from build123d import *

# Parameters (mm, degrees)
BOSS_EXTRUDE1_DEPTH = 19.5
BOSS_EXTRUDE5_DEPTH = 1.5
BOSS_EXTRUDE6_DEPTH = 1.5
SKETCH8_R           = 6.75
CUT_EXTRUDE2_DEPTH  = 35.70752685
BOSS_EXTRUDE7_DEPTH = 2.5
SKETCH10_R          = 1.75
BOSS_EXTRUDE8_DEPTH = 5
CHAMFER1_SIZE       = 1.5
SKETCH11_R          = 1.75
CUT_EXTRUDE3_DEPTH  = 3
CHAMFER2_SIZE       = 1
REVOLVE1_ANGLE      = 180


with BuildPart() as part:
    # Sketch1 → Boss-Extrude1 (new body)
    with BuildSketch(Plane.XY):
        Polygon((-11.779, -12.684829289), (-10.279, -12.684829289), (-10.279, -0.473504424), (-11.944063509, 0.487820441), (-11.944063509, 1.64252098), (-9.912974596, 2.815170711), (-9.427494989, 2.815170711), (-9.427494989, 4.973204454), (-6.75, 9.910826582), (0, 9.910826582), (0, 12.684829289), (-7.456216647, 12.684829289), (-13.444063509, 1.64252098), (-13.444063509, 0.487820441), align=None)
    extrude(amount=BOSS_EXTRUDE1_DEPTH)

    # Sketch6 → Boss-Extrude5 (add)
    with BuildSketch(Plane.XY.offset(19.5)):
        Polygon((0, 12.684829289), (-7.456216647, 12.684829289), (-13.444063509, 1.64252098), (-13.444063509, 0.487820441), (-11.779, -12.684829289), (0, -12.684829289), align=None)
    extrude(amount=-BOSS_EXTRUDE5_DEPTH)

    # Sketch7 → Boss-Extrude6 (add)
    with BuildSketch(Plane(origin=(0, 0, 0), x_dir=(-1, 0, 0), z_dir=(0, 0, -1))):
        Polygon((0, 12.684829289), (0, -12.684829289), (11.779, -12.684829289), (13.444063509, 0.487820441), (13.444063509, 1.64252098), (7.456216647, 12.684829289), align=None)
    extrude(amount=-BOSS_EXTRUDE6_DEPTH)

    # Sketch8 → Cut-Extrude2 (cut, through all)
    with BuildSketch(Plane(origin=(0, 12.684829289, 0), x_dir=(1, 0, 0), z_dir=(0, 1, 0))):
        with Locations((0, -9.75)):
            Circle(SKETCH8_R)
    extrude(amount=-CUT_EXTRUDE2_DEPTH, mode=Mode.SUBTRACT)

    # Sketch9 → Boss-Extrude7 (add, symmetric)
    with BuildSketch(Plane(origin=(0, 12.684829289, 0), x_dir=(1, 0, 0), z_dir=(0, 1, 0))):
        with BuildLine():
            Line((0, -1.5), (0, -3))
            ThreePointArc((0, -3), (-6.75, -9.75), (0, -16.5))
            Line((0, -16.5), (0, -18))
            ThreePointArc((0, -18), (-8.25, -9.75), (0, -1.5))
        make_face()
    extrude(amount=BOSS_EXTRUDE7_DEPTH, both=True)

    # Sketch10 → Boss-Extrude8 (add)
    with BuildSketch(Plane(origin=(0, 0, 0), x_dir=(0, 0, -1), z_dir=(1, 0, 0))):
        Polygon((-19.5, 12.684829289), (-27.043783602, 4.79693847), (-27.043783602, -4.79693847), (-19.5, -12.684829289), align=None)
        Polygon((-20.396891801, -1.659882024), (-20.396891801, 1.659882024), (-23.271891801, 3.319764048), (-26.146891801, 1.659882024), (-26.146891801, -1.659882024), (-23.271891801, -3.319764048), align=None, mode=Mode.SUBTRACT)
        Polygon((-23.271891801, -3.319764048), (-20.396891801, -1.659882024), (-20.396891801, 1.659882024), (-23.271891801, 3.319764048), (-26.146891801, 1.659882024), (-26.146891801, -1.659882024), align=None)
        with Locations(Location((-23.271891801, 0, 0), (0, 0, 90))):
            Circle(SKETCH10_R, mode=Mode.SUBTRACT)
        Polygon((7.543783602, 4.79693847), (0, 12.684829289), (0, -12.684829289), (7.543783602, -4.79693847), align=None)
        Polygon((6.646891801, 1.659882024), (3.771891801, 3.319764048), (0.896891801, 1.659882024), (0.896891801, -1.659882024), (3.771891801, -3.319764048), (6.646891801, -1.659882024), align=None, mode=Mode.SUBTRACT)
        Polygon((6.646891801, 1.659882024), (6.646891801, -1.659882024), (3.771891801, -3.319764048), (0.896891801, -1.659882024), (0.896891801, 1.659882024), (3.771891801, 3.319764048), align=None)
        with Locations(Location((3.771891801, 0, 0), (0, 0, 90))):
            Circle(SKETCH10_R, mode=Mode.SUBTRACT)
    extrude(amount=-BOSS_EXTRUDE8_DEPTH)

    # Chamfer1
    chamfer1_edges = [part.edges().sort_by_distance(p)[0] for p in [
        (-12.611531755, -6.098504424, 19.5),
        (-13.444063509, 1.065170711, 19.5),
        (-10.450140078, 7.163675135, 19.5),
        (-12.611531755, -6.098504424, 0),
        (-13.444063509, 1.065170711, 0),
        (-10.450140078, 7.163675135, 0),
    ]]
    chamfer(chamfer1_edges, length=CHAMFER1_SIZE)

    # Sketch11 → Cut-Extrude3 (cut)
    with BuildSketch(Plane.ZY.offset(5)):
        Polygon((-6.646891801, 1.659882024), (-3.771891801, 3.319764048), (-0.896891801, 1.659882024), (-0.896891801, -1.659882024), (-3.771891801, -3.319764048), (-6.646891801, -1.659882024), align=None)
        with Locations(Location((-3.771891801, 0, 0), (0, 0, 90))):
            Circle(SKETCH11_R, mode=Mode.SUBTRACT)
        Polygon((20.396891801, 1.659882024), (23.271891801, 3.319764048), (26.146891801, 1.659882024), (26.146891801, -1.659882024), (23.271891801, -3.319764048), (20.396891801, -1.659882024), align=None)
        with Locations(Location((23.271891801, 0, 0), (0, 0, 90))):
            Circle(SKETCH11_R, mode=Mode.SUBTRACT)
    extrude(amount=-CUT_EXTRUDE3_DEPTH, mode=Mode.SUBTRACT)

    # Chamfer2
    chamfer2_edges = [part.edges().sort_by_distance(p)[0] for p in [
        (-8.25, 15.184829289, 9.75),
    ]]
    chamfer(chamfer2_edges, length=CHAMFER2_SIZE)

    # Sketch12 → Revolve1 (revolve)
    with BuildSketch(Plane(origin=(0, 0, 0), x_dir=(0, 0, -1), z_dir=(1, 0, 0))):
        Polygon((-16.5, 15.184829289), (-16.5, 14.184829289), (-15.75, 14.684829289), align=None)
    revolve(axis=Axis((0, 15.184829289, 9.75), (0, -1, 0)), revolution_arc=REVOLVE1_ANGLE)


solid = part.part
Geometry check sheet. Reference: the model listing, model coordinates, mm. A direction names the side the tool comes from. Coordinates: 2 decimals unless noted, no trailing zeros. Order: outer loops, then holes, each group sorted by start corner. A loop starts at its lowest first (then second) coordinate and runs counter-clockwise, first axis right, second up. Notation, with made-up numbers: (55.25, -9.5) -> (64.25, -9.5) arc R37 ccw to (64.25, 29.5) -> close; hole circle Ø4 at (88, 8.25). An arc over 180 degrees is marked (long way). Use a Markdown table: item, result. Add a question column.
1. Go/stop test with flat-tipped pins: pin 1 Ø8.5 at (y, z) = (2, 24) entering from -X; pin 2 Ø6.5 at (y, z) = (-1, -3) entering from -X; pin 3 Ø5 at (y, z) = (11.5, 10.5) entering from +X. Record where each tip stops, or that it passes through.
2. Cross-section at A-A (y = 0). Give the number of separate pieces and of enclosed holes in the cut face, and give its area (3 significant figures).
3. Cross-section at D-D (y = -5.25). Enter the section's corners in (x, z).
4. Mould release check, pull along Z, two halves, no side actions. Record for faces 6 (the face through (-2.46, 8.69, -3.82)), 7 (the face through (-0.986, -0.228, -2.037)), 8 (the face through (-5, 12.685, 18)): pulls with the +Z half, pulls with the -Z half, needs draft (parallel to the pull), parting line crosses it, or undercut.
5. Cross-section at B-B (z = 24). Enter the section's corners in (x, y), and give its area (3 significant figures).
6. Material ranges on L1, parallel to Z at x = -1.05, y = 0; L2, parallel to Z at x = -7.5, y = 2; L3, parallel to Z at x = -2.25, y = -2.5, recorded low to high.
7. Set-up check for faces 1 (the face through (-5, 0.2, -0.4)), 2 (the face through (-4, 0, 26.147)), 3 (the face through (-5, 0, 20)), 4 (the face through (-2.46, -8.69, 23.32)), 5 (the face through (-8.107, 7.407, 9.634)): record each of +Z, -Z, +X, -X, +Y, -Y from which the full face is reachable in a straight line by a thin tool's end or side.
Filled sheet:
| question | item | result |
|---|---|---|
| 1 | pin 1 | x = -5 |
| 1 | pin 2 | x = -12.02 |
| 1 | pin 3 | x = -5.92 |
| 2 | separate pieces | 3 |
| 2 | enclosed holes | 0 |
| 2 | area | 102 mm2 |
| 3 | outline | (-12.72, 1.5) -> (-11.21, 0) -> (-5, 0) -> (-5, -7.11) -> (0, -7.11) -> (0, 1.5) -> (-10.28, 1.5) -> (-10.28, 18) -> (0, 18) -> (0, 26.61) -> (-5, 26.61) -> (-5, 19.5) -> (-11.21, 19.5) -> (-12.72, 18) -> close |
| 4 | face 6 | pulls with the -Z half |
| 4 | face 7 | undercut |
| 4 | face 8 | needs draft |
| 5 | outline | (-5, -7.98) -> (0, -7.98) -> (0, -1.59) -> (-2, -1.59) -> (-2, -2.9) -> (-5, -2.9) -> close; (-5, 2.9) -> (-2, 2.9) -> (-2, 1.59) -> (0, 1.59) -> (0, 7.98) -> (-5, 7.98) -> close |
| 5 | area | 56.0 mm2 |
| 6 | L1 | -7.54 to -5.52, -2.02 to 1.5, 18 to 21.52, 25.02 to 27.04 |
| 6 | L2 | 0 to 1.5, 18 to 19.5 |
| 6 | L3 | -7.54 to -5.19, -2.35 to 1.5, 18 to 21.85, 24.69 to 27.04 |
| 7 | face 1 | -Z, -X, +Y, -Y |
| 7 | face 2 | -X |
| 7 | face 3 | +Z, -X, +Y, -Y |
| 7 | face 4 | +Z, +X, -X, -Y |
| 7 | face 5 | +X, -Y |
